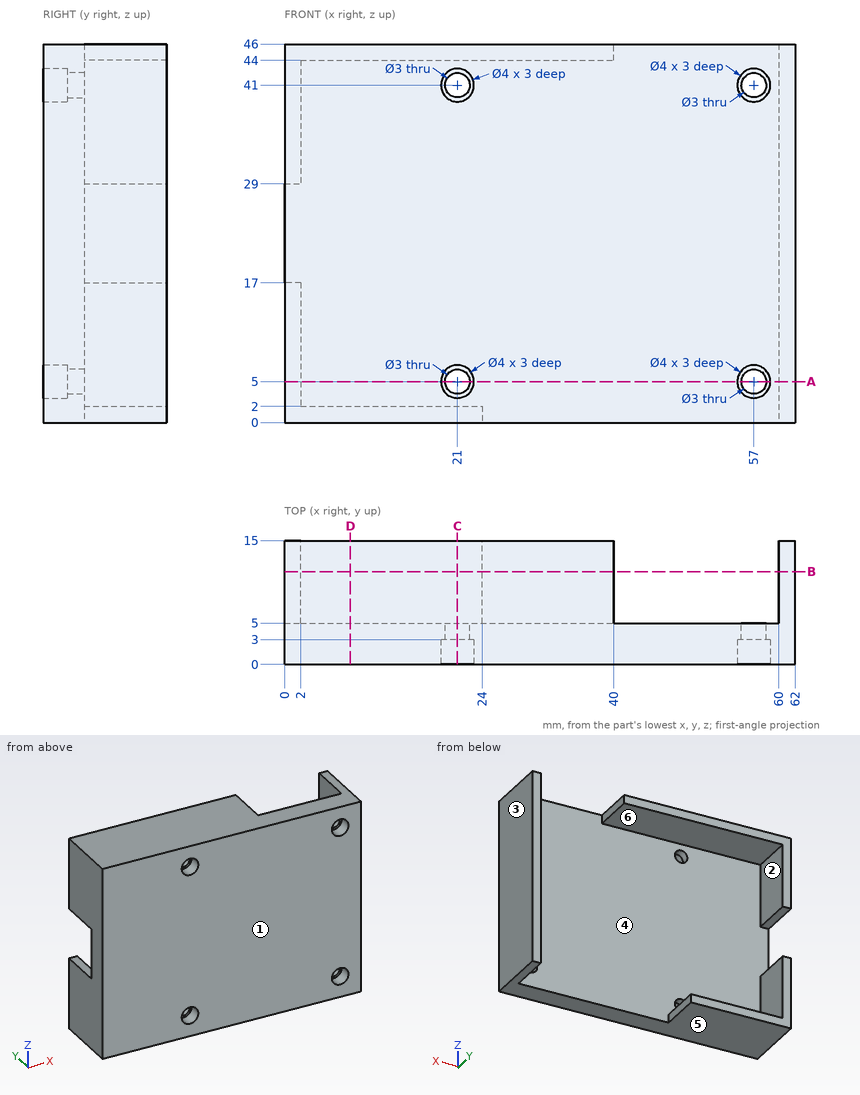
Print and shaded views of the part. All mm, measured from the part's lowest x, y and z. A direction names the side the tool comes from. Give positions to 0.01 mm unless a question says otherwise; leave off trailing zeros. Loops run counter-clockwise (first coordinate to the right, second up) from the corner with the lowest first, then second, coordinate; pieces in that order, holes last. Notation, with made-up numbers: (12, 88.5) - (61, 88.5) arc R18 ccw to (61, 117.5) - close; hole circle Ø1 at (18.25, -20). An arc over 180 degrees is marked (long way). Use a Markdown table: item, result.
(1) Drop flat-ended pins along their axis: pin 1 Ø3 at (x, z) = (20.5, 4.5) entering from -Y; pin 2 Ø5 at (x, z) = (57, 5) entering from +Y; pin 3 Ø1.5 at (y, z) = (7, 20) entering from -X. Give the stop position or say it passes through.
Taken from the geometry:
| item | result |
|---|---|
| pin 1 | y = 0 |
| pin 2 | y = 5 |
| pin 3 | x = 60 |
(2) Band-saw the part on B-B (y = 11.25). Give the cut face in (x, z).
Taken from the geometry:
| item | result |
|---|---|
| outline | (0, 0) - (24, 0) - (24, 2) - (2, 2) - (2, 17) - (0, 17) - close; (0, 29) - (2, 29) - (2, 44) - (40, 44) - (40, 46) - (0, 46) - close; (60, 0) - (62, 0) - (62, 46) - (60, 46) - close |
(3) Band-saw the part on C-C (x = 21). Give the cut face in (y, z), and give its area (3 significant figures).
Taken from the geometry:
| item | result |
|---|---|
| outline | (0, 0) - (15, 0) - (15, 2) - (5, 2) - (5, 3.5) - (3, 3.5) - (3, 3) - (0, 3) - close; (0, 7) - (3, 7) - (3, 6.5) - (5, 6.5) - (5, 39.5) - (3, 39.5) - (3, 39) - (0, 39) - close; (0, 43) - (3, 43) - (3, 42.5) - (5, 42.5) - (5, 44) - (15, 44) - (15, 46) - (0, 46) - close |
| area | 234 mm2 |
(4) Which spindle directions (+Z, -Z, +X, -X, +Y, -Y) get a long thin tool onto all of the face, cutting with end or side? Do the marked faces 1 and 2. Say none if no direction does.
Taken from the geometry:
| item | result |
|---|---|
| face 1 | +Z, -Z, +X, -X, -Y |
| face 2 | +Y |
(5) Wall check: line 1 along X through (y, z) = (3.9, 5); line 2 along X through (y, z) = (1.45, 5); line 3 along Z through (x, y) = (14, 7.5). Give the ranges that are in metal, low to high.
Taken from the geometry:
| item | result |
|---|---|
| line 1 | 0 to 19.5, 22.5 to 55.5, 58.5 to 62 |
| line 2 | 0 to 19, 23 to 55, 59 to 62 |
| line 3 | 0 to 2, 44 to 46 |
(6) Pull direction Z, two halves, no side cores. Call the marked faces 3, 4, 5 and 6: +Z half, -Z half, draft (parallel to the pull), parting line (faces both ways), or undercut.
Taken from the geometry:
| item | result |
|---|---|
| face 3 | draft |
| face 4 | undercut |
| face 5 | -Z half |
| face 6 | undercut |
(7) Band-saw the part on A-A (z = 5). Give the cut face in (x, y), and give its area (3 significant figures).
Taken from the geometry:
| item | result |
|---|---|
| outline | (0, 0) - (19, 0) - (19, 3) - (19.5, 3) - (19.5, 5) - (2, 5) - (2, 15) - (0, 15) - close; (22.5, 3) - (23, 3) - (23, 0) - (55, 0) - (55, 3) - (55.5, 3) - (55.5, 5) - (22.5, 5) - close; (58.5, 3) - (59, 3) - (59, 0) - (62, 0) - (62, 15) - (60, 15) - (60, 5) - (58.5, 5) - close |
| area | 314 mm2 |
(8) Band-saw the part on D-D (x = 8). Give the cut face in (y, z), and give its area (3 significant figures).
Taken from the geometry:
| item | result |
|---|---|
| outline | (0, 0) - (15, 0) - (15, 2) - (5, 2) - (5, 44) - (15, 44) - (15, 46) - (0, 46) - close |
| area | 270 mm2 |
